Could you check a few things on this drawing? It's one solid part, dimensions in mm from its lowest x, y, z. A direction names the side the tool comes from. Coordinates: 2 decimals unless noted, no trailing zeros. Order: outer loops, then holes, each group sorted by start corner. A loop starts at its lowest first (then second) coordinate and runs counter-clockwise, first axis right, second up.
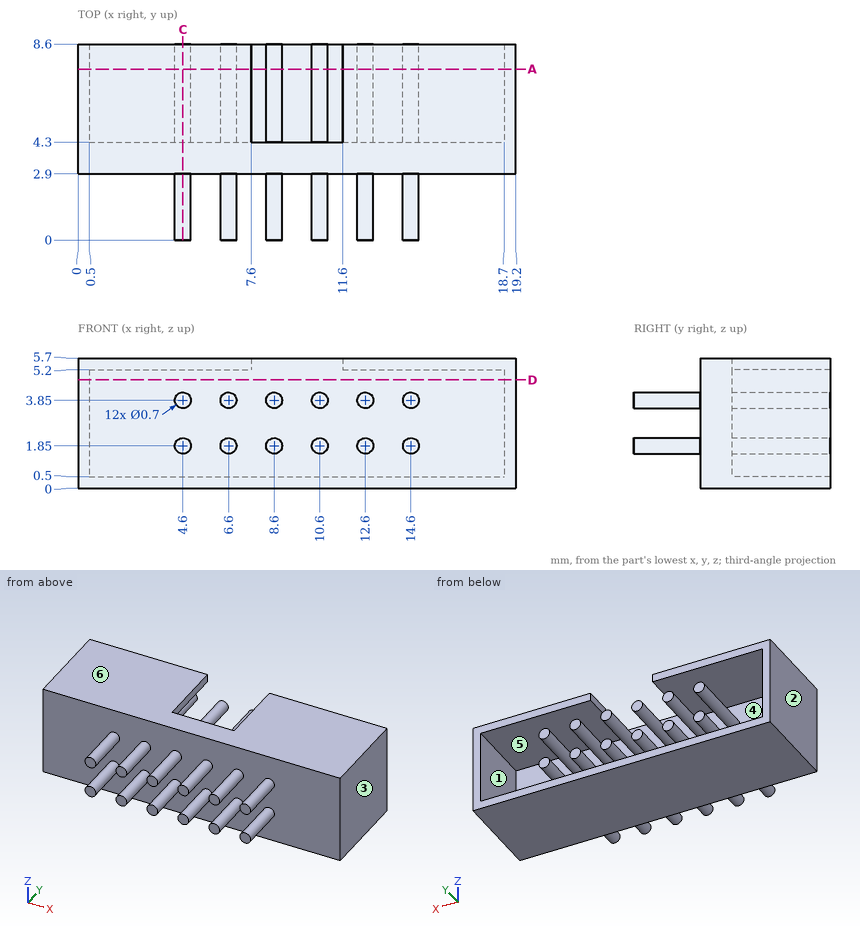
1. On a 3-axis mill with a long thin cutter (end or side, diameter ignored), from which of +Z, -Z, +X, -X, +Y, -Y can I reach the whole of each face in a straight line? I mean the marked faces 5 and 6. Say none if no direction works.
Completed:
face 5: +Y
face 6: +Z, +X, -X, +Y, -Y
2. Imagine slicing it at A-A on y = 7.5. Give the number of separate pieces and of enclosed holes in the cut face, then the cut area to 3 significant figures.
Completed:
separate pieces: 13
enclosed holes: 0
area: 26.5 mm2
3. Imagine slicing it at C-C on x = 4.6. Please give me the cut outline in (y, z).
Completed:
outline: (0, 1.5) - (2.9, 1.5) - (2.9, 0) - (8.6, 0) - (8.6, 0.5) - (4.3, 0.5) - (4.3, 1.5) - (8.6, 1.5) - (8.6, 2.2) - (4.3, 2.2) - (4.3, 3.5) - (8.6, 3.5) - (8.6, 4.2) - (4.3, 4.2) - (4.3, 5.2) - (8.6, 5.2) - (8.6, 5.7) - (2.9, 5.7) - (2.9, 4.2) - (0, 4.2) - (0, 3.5) - (2.9, 3.5) - (2.9, 2.2) - (0, 2.2) - close
4. Thinking about a two-plate mould opening in X: for the marked faces 1, 2, 3 and 4, which applies, pulls with the +X half, pulls with the -X half, needs draft (parallel to the pull), parting line crosses it, or undercut?
Completed:
face 1: undercut
face 2: pulls with the -X half
face 3: pulls with the +X half
face 4: undercut
5. I'm going to push a flat-ended pin straight in: pin 1 (4.5 mm diameter, centred on x = 3.5, y = 5.5, fed in from -Z). Where does the tip first touch, or does it pass through?
Completed:
pin 1: stops at z = 0
6. Imagine slicing it at D-D on z = 4.75. Please give me the cut outline in (x, y).
Completed:
outline: (0, 2.9) - (19.2, 2.9) - (19.2, 8.6) - (18.7, 8.6) - (18.7, 4.3) - (0.5, 4.3) - (0.5, 8.6) - (0, 8.6) - close
7. Please list where these lines run through material, in increasing order: probe 1 along X at (y, z) = (7.25, 1.3); probe 2 along Z at (x, y) = (15.75, 7); probe 3 along X at (y, z) = (1.25, 1.8).
Completed:
probe 1: x = 0 to 0.5, 18.7 to 19.2
probe 2: z = 0 to 0.5, 5.2 to 5.7
probe 3: x = 4.25 to 4.95, 6.25 to 6.95, 8.25 to 8.95, 10.25 to 10.95, 12.25 to 12.95, 14.25 to 14.95
